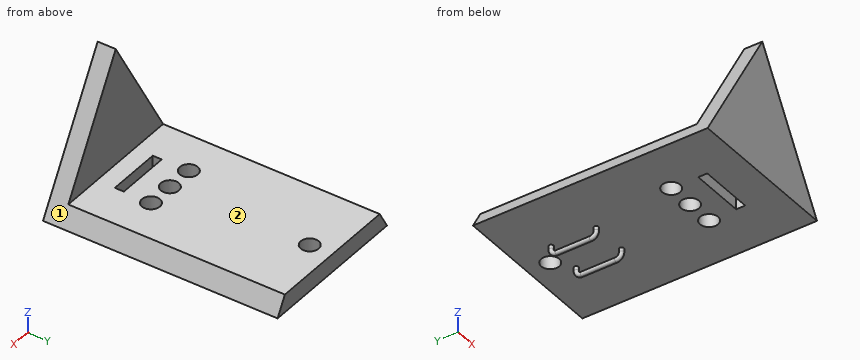
```python
from build123d import *

# Parameters (mm, degrees)
MAIN_FRAME_DEPTH     = 130
SHELL1_T             = -10
CUT_EXTRUDE1_DEPTH   = 174.277234512
EXTERNAL_PORTS_REACH = 158.205
SKETCH5_R            = 5
SKETCH5_W            = 30
SKETCH5_H            = 5
SKETCH7_R            = 1.25


with BuildPart() as part:
    # Sketch1 → Main Frame (new body)
    with BuildSketch(Plane(origin=(0, 0, 0), x_dir=(1, 0, 0), z_dir=(0, 1, 0))):
        Polygon((86.602540378, 0), (43.301270189, 75), (-43.301270189, 75), (-86.602540378, 0), (-43.301270189, -75), (43.301270189, -75), align=None)
    extrude(amount=MAIN_FRAME_DEPTH)

    # Shell1
    shell1_openings = [part.faces().sort_by_distance(p)[0] for p in [
        (0, 130, 0),
    ]]
    offset(amount=SHELL1_T, openings=shell1_openings, kind=Kind.INTERSECTION)

    # Sketch2 → Cut-Extrude1 (cut, through all)
    with BuildSketch(Plane(origin=(0, 130, 0), x_dir=(1, 0, 0), z_dir=(0, 1, 0))):
        Polygon((-43.301270189, 75), (0, 0), (43.301270189, 75), (86.602540378, 0), (43.301270189, -75), (-43.301270189, -75), (-86.602540378, 0), align=None)
    extrude(amount=-CUT_EXTRUDE1_DEPTH, mode=Mode.SUBTRACT)

    # Sketch5 → External Ports (cut, up to next)
    with BuildSketch(Plane(origin=(0, 0, -75), x_dir=(-1, 0, 0), z_dir=(0, 0, -1)), mode=Mode.PRIVATE) as external_ports_sk1:
        with Locations((-15, 40)):
            Circle(SKETCH5_R)
    external_ports_tool1 = extrude(external_ports_sk1.sketch, amount=-EXTERNAL_PORTS_REACH, mode=Mode.PRIVATE) & part.part
    # Sketch5 → External Ports (cut, up to next)
    with BuildSketch(Plane(origin=(0, 0, -75), x_dir=(-1, 0, 0), z_dir=(0, 0, -1)), mode=Mode.PRIVATE) as external_ports_sk2:
        with Locations((0, 40)):
            Circle(SKETCH5_R)
    external_ports_tool2 = extrude(external_ports_sk2.sketch, amount=-EXTERNAL_PORTS_REACH, mode=Mode.PRIVATE) & part.part
    # Sketch5 → External Ports (cut, up to next)
    with BuildSketch(Plane(origin=(0, 0, -75), x_dir=(-1, 0, 0), z_dir=(0, 0, -1)), mode=Mode.PRIVATE) as external_ports_sk3:
        with Locations((15, 40)):
            Circle(SKETCH5_R)
    external_ports_tool3 = extrude(external_ports_sk3.sketch, amount=-EXTERNAL_PORTS_REACH, mode=Mode.PRIVATE) & part.part
    # Sketch5 → External Ports (cut, up to next)
    with BuildSketch(Plane(origin=(0, 0, -75), x_dir=(-1, 0, 0), z_dir=(0, 0, -1)), mode=Mode.PRIVATE) as external_ports_sk4:
        with Locations((0, 117.5)):
            Circle(SKETCH5_R)
    external_ports_tool4 = extrude(external_ports_sk4.sketch, amount=-EXTERNAL_PORTS_REACH, mode=Mode.PRIVATE) & part.part
    # Sketch5 → External Ports (cut, up to next)
    with BuildSketch(Plane(origin=(0, 0, -75), x_dir=(-1, 0, 0), z_dir=(0, 0, -1)), mode=Mode.PRIVATE) as external_ports_sk5:
        with Locations((0, 22.5)):
            Rectangle(SKETCH5_W, SKETCH5_H)
    external_ports_tool5 = extrude(external_ports_sk5.sketch, amount=-EXTERNAL_PORTS_REACH, mode=Mode.PRIVATE) & part.part
    add(external_ports_tool1.solids().sort_by_distance((15, 40, -75))[0], mode=Mode.SUBTRACT)
    add(external_ports_tool2.solids().sort_by_distance((0, 40, -75))[0], mode=Mode.SUBTRACT)
    add(external_ports_tool3.solids().sort_by_distance((-15, 40, -75))[0], mode=Mode.SUBTRACT)
    add(external_ports_tool4.solids().sort_by_distance((0, 117.5, -75))[0], mode=Mode.SUBTRACT)
    add(external_ports_tool5.solids().sort_by_distance((0, 22.5, -75))[0], mode=Mode.SUBTRACT)

    # Boom Mount: sweep along a path in Sketch6
    with BuildLine(Plane(origin=(10, 0, 0), x_dir=(0, 0, -1), z_dir=(1, 0, 0))) as boom_mount_path:
        Line((75, 110), (77, 110))
        ThreePointArc((77, 110), (79.121320344, 109.121320344), (80, 107))
        Line((80, 107), (80, 88))
        ThreePointArc((80, 88), (79.121320344, 85.878679656), (77, 85))
        Line((77, 85), (75, 85))
    # Sketch7 → Boom Mount (sweep)
    with BuildSketch(Plane(origin=(0, 0, -75), x_dir=(-1, 0, 0), z_dir=(0, 0, -1))):
        with Locations((-10, 110)):
            Circle(SKETCH7_R)
    boom_mount = sweep(path=boom_mount_path.line)

    # Mirror1: Boom Mount across plane
    add(boom_mount.mirror(Plane(origin=(0, 0, 0), x_dir=(0, 0, 1), z_dir=(1, 0, 0))))


solid = part.part
```
Check sheet for the modelled part. Datum: model origin and axes. Units: mm. Face numbers are marked on the shaded views. A direction names the side the tool comes from. Coordinates: 2 decimals unless noted, no trailing zeros. Loops run counter-clockwise (first coordinate to the right, second up) from the corner with the lowest first, then second, coordinate; pieces in that order, holes last.
1) Gauge pin test, flat ends, axial feed: pin 1 (13 mm diameter, centred on x = -15, y = 40, fed in from +Z); pin 2 (1 mm diameter, centred on y = 21.5, z = -71.5, fed in from +X); pin 3 (12 mm diameter, centred on x = -26.5, z = -29, fed in from -Y); pin 4 (4 mm diameter, centred on x = 6.5, z = -58.5, fed in from +Y). Record the tip position at first contact, or that the pin passes through.
2) Sectioned sample at A-A (y = 40). Record the boundary of the cut face in (x, z), and give its area (3 significant figures).
3) Sectioned sample at C-C (x = 29). Record the boundary of the cut face in (y, z).
4) Material ranges on probe 1 along Z at (x, y) = (2, 29.5); probe 2 along Y at (x, z) = (12, -35); probe 3 along Z at (x, y) = (-11, 89.5), recorded low to high.
5) Sectioned sample at D-D (z = -30). Record the boundary of the cut face in (x, y), and give its area (3 significant figures).
6) Access from +Z, -Z, +X, -X, +Y, -Y to the whole of each face (thin tool, end or side, straight path). Record for the marked faces 1 and 2.
7) Sectioned sample at B-B (y = 117.5). Record the boundary of the cut face in (x, z), and give its area (3 significant figures).
Check sheet entries:
1. pin 1: stops at z = -65
1. pin 2: stops at x = 41.57
1. pin 3: passes through
1. pin 4: stops at y = 10
2. outline: (-43.3, -75) - (-20, -75) - (-20, -65) - (-37.53, -65) - close; (-10, -75) - (-5, -75) - (-5, -65) - (-10, -65) - close; (5, -75) - (10, -75) - (10, -65) - (5, -65) - close; (20, -75) - (43.3, -75) - (37.53, -65) - (20, -65) - close
2. area: 508 mm2
3. outline: (0, -75) - (130, -75) - (130, -65) - (10, -65) - (10, -50.23) - (0, -50.23) - close
4. probe 1: z = -75 to -65
4. probe 2: y = 0 to 10
4. probe 3: z = -80.75 to -79.25, -75 to -65
5. outline: (-17.32, 0) - (17.32, 0) - (17.32, 10) - (-17.32, 10) - close
5. area: 346 mm2
6. face 1: +Z, +X, +Y, -Y
6. face 2: +Z, +X, -X, +Y
7. outline: (-43.3, -75) - (-5, -75) - (-5, -65) - (-37.53, -65) - close; (5, -75) - (43.3, -75) - (37.53, -65) - (5, -65) - close
7. area: 708 mm2
